Could you check a few things on this model? Use its own coordinates, in mm. A direction names the side the tool comes from. Give positions to 0.01 mm unless a question says otherwise; leave off trailing zeros. Order: outer loops, then holes, each group sorted by start corner. A loop starts at its lowest first (then second) coordinate and runs counter-clockwise, first axis right, second up. Notation, with made-up numbers: M 41.25,58.25 L 55.25,58.25 A20 ccw 55.25,79.25 Z; hole C 78.25,52.25 d2. An arc over 180 degrees is marked long. Return JSON: item names as keys, results as strings. Group by question number.
```python
from build123d import *

# Parameters (mm, degrees)
SK_SHANK_R        = 2.5
EXT_SHANK_DEPTH   = 25
SK_HEAD_R         = 4.25
EXT_HEAD_DEPTH    = 5
CUT_HEX_DEPTH     = 3
CHAMFER_HEAD_SIZE = 0.4


with BuildPart() as part:
    # Sk_shank → Ext_shank (new body)
    with BuildSketch(Plane.XY):
        Circle(SK_SHANK_R)
    extrude(amount=EXT_SHANK_DEPTH)

    # Sk_head → Ext_head (add)
    with BuildSketch(Plane.XY):
        Circle(SK_HEAD_R)
    extrude(amount=EXT_HEAD_DEPTH)

    # Sk_hex → Cut_hex (cut)
    with BuildSketch(Plane.XY):
        Polygon((2.309401077, 0), (1.154700538, 2), (-1.154700538, 2), (-2.309401077, 0), (-1.154700538, -2), (1.154700538, -2), align=None)
    extrude(amount=CUT_HEX_DEPTH, mode=Mode.SUBTRACT)

    # Chamfer_head
    chamfer_head_edges = [part.edges().sort_by_distance(p)[0] for p in [
        (1.732050808, -1, 0),
        (1.732050808, 1, 0),
        (0, 2, 0),
        (-1.732050808, 1, 0),
        (-1.732050808, -1, 0),
        (0, -2, 0),
        (-4.25, 0, 0),
    ]]
    chamfer(chamfer_head_edges, length=CHAMFER_HEAD_SIZE)


solid = part.part
```
1. I need wall thicknesses on L1, parallel to Z at x = -0.25, y = 3.5; L2, parallel to Z at x = 1.25, y = 1.75; L3, parallel to X at y = 1.5, z = 2.25. Which ranges of each line are inside material? Lowest first, please. Write a range as from..to.
2. Imagine slicing it at C-C, the plane z = 17.25. Please give me the cut outline in (x, y), plus the area to 3 significant figures.
3. For pin 1 (0.7 mm diameter, centred on x = -0.5, z = 1.5, fed in from -Y); pin 2 (1 mm diameter, centred on y = 1, z = 10, fed in from +X); pin 3 (3 mm diameter, centred on x = 1.5, z = 14, fed in from -Y), each with a flat end and sliding along its axis, tell me the tip position at first contact or that it passes through.
4. If we mould it in two halves opening along X, with no side actions, what happens to faces 1 (the flat face through (1.913, 1.082, 0.203)), 2 (the cylindrical face through (-0.54, -2.44, 14.86)), 3 (the flat face through (0, -3, 0))? For each: pulls with the +X half, pulls with the -X half, needs draft (parallel to the pull), parting line crosses it, or undercut.
5. Which directions (+Z, -Z, +X, -X, +Y, -Y) give clear straight access to the entire face, cutting with the end or side of a thin tool? Please do faces 4 (the flat face through (2, -2, 5)), 5 (the flat face through (0, 0, 25)), 6 (the flat face through (1.74, 0.99, 1.68)).
6. Imagine slicing it at A-A, the plane z = 2.75. Please give me the cut outline in (x, y).
7. Imagine slicing it at B-B, the plane x = 0. Please give me the cut outline in (y, z).
Values:
{
 "1": {"L1": "z = 0..5", "L2": "z = 3..25", "L3": "x = -3.98..-1.44, 1.44..3.98"},
 "2": {"outline": "C 0,0 d5", "area": "19.6 mm²"},
 "3": {"pin 1": "stops at y = -4.25", "pin 2": "stops at x = 2.45", "pin 3": "stops at y = -2.5"},
 "4": {"face 1": "undercut", "face 2": "parting line crosses it", "face 3": "needs draft"},
 "5": {"face 4": "+Z", "face 5": "+Z, +X, -X, +Y, -Y", "face 6": "-Z"},
 "6": {"outline": "C 0,0 d8.5; hole M -2.31,0 L -1.15,-2 L 1.15,-2 L 2.31,0 L 1.15,2 L -1.15,2 Z"},
 "7": {"outline": "M -4.25,0.4 L -3.85,0 L -2.4,0 L -2,0.4 L -2,3 L 2,3 L 2,0.4 L 2.4,0 L 3.85,0 L 4.25,0.4 L 4.25,5 L 2.5,5 L 2.5,25 L -2.5,25 L -2.5,5 L -4.25,5 Z"}
}
